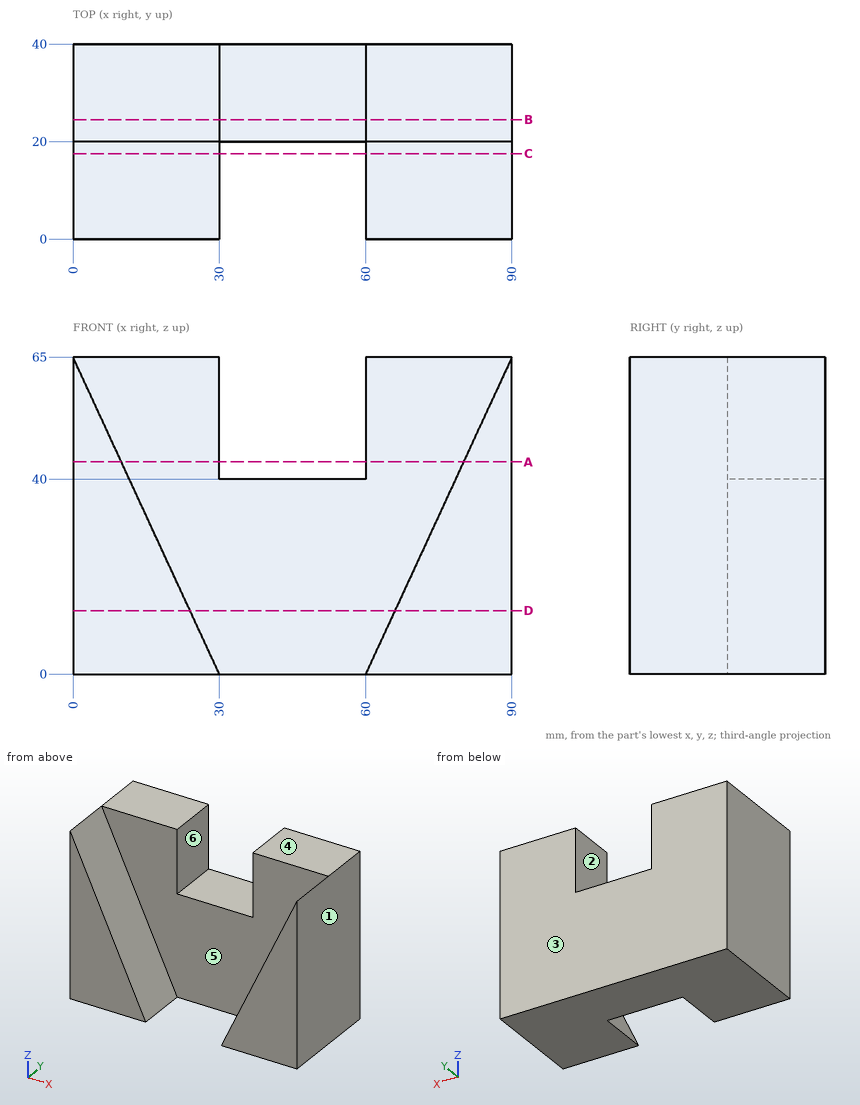
Verification items for this drawing (mm, ordinates from the low corner). A direction names the side the tool comes from. Give positions to 0.01 mm unless a question says otherwise; leave off trailing zeros. Write each loop counter-clockwise with the first axis right and the second up, starting at its lowest first coordinate (ties: lowest second). Pieces come first, ordered by that corner, then holes. Notation, with made-up numbers: (59.25, 86) - (92.25, 86) arc R13 cw to (92.25, 109) - close; hole circle Ø4 at (-20, 64). An arc over 180 degrees is marked (long way). Answer as a JSON object with one key per item and string values. Group by question number.
1) Sectioned sample at B-B (y = 24.5). Record the cut outline in (x, z).
2) Sectioned sample at A-A (z = 43.5). Record the cut outline in (x, y).
3) Thickness scan on probe 1 along Y at (x, z) = (79.5, 46); probe 2 along X at (y, z) = (11, 10.5); probe 3 along X at (y, z) = (15, 15.5). Record the ranges inside material, lowest first. Write a range as from..to.
4) Access from +Z, -Z, +X, -X, +Y, -Y to the whole of each face (thin tool, end or side, straight path). Record for the marked faces 4, 5 and 6.
5) Release check for a two-part mould opening along X. For the marked faces 1, 2 and 3 record: pulls with the +X half, pulls with the -X half, needs draft (parallel to the pull), parting line crosses it, or undercut.
6) Sectioned sample at C-C (y = 17.5). Record the cut outline in (x, z), then the cut area to 3 significant figures.
7) Depth check by flat-ended pin: P1, Ø6, axis at x = 38.5, y = 33.5, coming from the +Z side. Enter the tip coordinate at first touch or a pass-through.
8) Sectioned sample at D-D (z = 13). Record the cut outline in (x, y), then the cut area to 3 significant figures.
Geometry results:
{
 "1": {"outline": "(0, 0) - (90, 0) - (90, 65) - (60, 65) - (60, 40) - (30, 40) - (30, 65) - (0, 65) - close"},
 "2": {"outline": "(0, 0) - (9.92, 0) - (9.92, 20) - (30, 20) - (30, 40) - (0, 40) - close; (60, 20) - (80.08, 20) - (80.08, 0) - (90, 0) - (90, 40) - (60, 40) - close"},
 "3": {"probe 1": "y = 20..40", "probe 2": "x = 0..25.15, 64.85..90", "probe 3": "x = 0..22.85, 67.15..90"},
 "4": {"face 4": "+Z, +X, -X, +Y, -Y", "face 5": "+Z, -Y", "face 6": "+Z, +Y, -Y"},
 "5": {"face 1": "pulls with the +X half", "face 2": "undercut", "face 3": "needs draft"},
 "6": {"outline": "(0, 0) - (30, 0) - (0, 65) - close; (60, 0) - (90, 0) - (90, 65) - close", "area": "1,950 mm^2"},
 "7": {"P1": "stops at z = 40"},
 "8": {"outline": "(0, 0) - (24, 0) - (24, 20) - (66, 20) - (66, 0) - (90, 0) - (90, 40) - (0, 40) - close", "area": "2,760 mm^2"}
}
